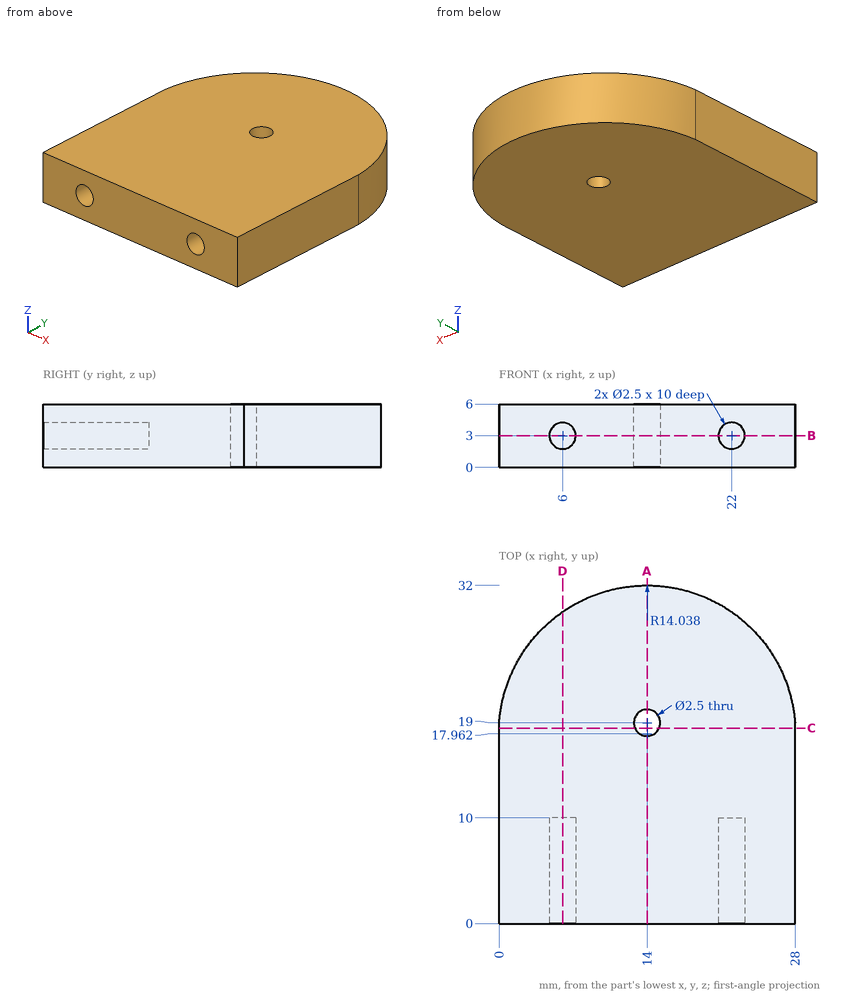
Geometry check sheet. Reference: drawing and pictorial views, mm from the part's lowest x, y, z. Give positions to 0.01 mm unless a question says otherwise; leave off trailing zeros. Order: outer loops, then holes, each group sorted by start corner. A loop starts at its lowest first (then second) coordinate and runs counter-clockwise, first axis right, second up. Notation, with made-up numbers: (-37, 41.25) - (-5, 41.25) arc R32 cw to (-5, 79.25) - close; hole circle Ø7 at (59, 17.25). An arc over 180 degrees is marked (long way). Answer as CSV lines item,"result". Start each with the question number.
Item 1: Section check C-C, the plane y = 18.5. Record the boundary of the cut face in (x, z) (1 decimal).
Item 2: Section check B-B, the plane z = 3. Record the boundary of the cut face in (x, y).
Item 3: Material ranges on L1, parallel to X at y = 3.5, z = 3; L2, parallel to X at y = 7.5, z = 3.65; L3, parallel to Y at x = 14, z = 2.9, recorded low to high.
Item 4: Section check A-A, the plane x = 14. Record the boundary of the cut face in (y, z).
Item 5: Gauge pin test, flat ends, axial feed: pin 1 (6 mm diameter, centred on x = 16.5, y = 10.5, fed in from -Z); pin 2 (0.8 mm diameter, centred on x = 22, z = 3, fed in from -Y); pin 3 (3 mm diameter, centred on x = 22, z = 3, fed in from +Y) (1 decimal). Record the tip position at first contact, or that the pin passes through.
Item 6: Section check D-D, the plane x = 6. Record the boundary of the cut face in (y, z).
Filled in:
1,outline,"(0, 0) - (12.9, 0) - (12.9, 6) - (0, 6) - close; (15.1, 0) - (28, 0) - (28, 6) - (15.1, 6) - close"
2,outline,"(0, 0) - (4.75, 0) - (4.75, 10) - (7.25, 10) - (7.25, 0) - (20.75, 0) - (20.75, 10) - (23.25, 10) - (23.25, 0) - (28, 0) - (28, 19) arc R14.04 ccw to (0, 19) - close; hole circle Ø2.5 at (14, 19)"
3,L1,"0 to 4.75, 7.25 to 20.75, 23.25 to 28"
3,L2,"0 to 4.93, 7.07 to 20.93, 23.07 to 28"
3,L3,"0 to 17.75, 20.25 to 32"
4,outline,"(0, 0) - (17.75, 0) - (17.75, 6) - (0, 6) - close; (20.25, 0) - (32, 0) - (32, 6) - (20.25, 6) - close"
5,pin 1,"z = 0"
5,pin 2,"y = 10"
5,pin 3,"y = 30.4"
6,outline,"(0, 0) - (29.5, 0) - (29.5, 6) - (0, 6) - (0, 4.25) - (10, 4.25) - (10, 1.75) - (0, 1.75) - close"
